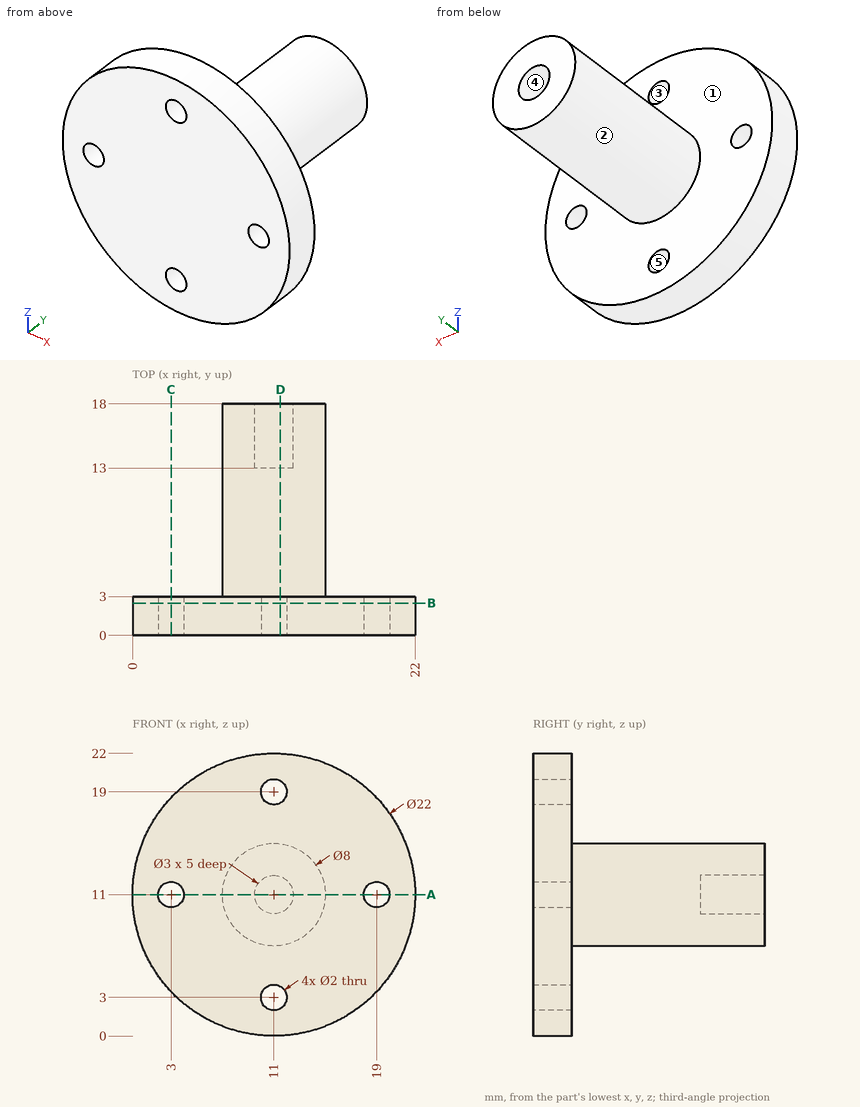
Check sheet for the drawn part. Datum: minimum x, y, z corner. Units: mm. A direction names the side the tool comes from. Round coordinates to 2 decimals unless told otherwise and drop trailing zeros. Loops run counter-clockwise (first coordinate to the right, second up) from the corner with the lowest first, then second, coordinate; pieces in that order, holes last. Notation, with made-up numbers: (7.5, 35) - (63.5, 35) arc R32 cw to (63.5, 67) - close; hole circle Ø5 at (-28.5, -36.75). An arc over 180 degrees is marked (long way). Use one line per item in the form item = value.
1. Section check B-B on y = 2.5. Record the cut outline in (x, z).
A:
outline = circle Ø22 at (11, 11); hole circle Ø2 at (3, 11); hole circle Ø2 at (11, 3); hole circle Ø2 at (11, 19); hole circle Ø2 at (19, 11)
2. Section check C-C on x = 3. Record the cut outline in (y, z), and give its area (3 significant figures).
A:
outline = (0, 3.45) - (3, 3.45) - (3, 10) - (0, 10) - close; (0, 12) - (3, 12) - (3, 18.55) - (0, 18.55) - close
area = 39.3 mm²
3. Section check D-D on x = 11.5. Record the cut outline in (y, z), and give its area (3 significant figures).
A:
outline = (0, 0.01) - (3, 0.01) - (3, 2.13) - (0, 2.13) - close; (0, 3.87) - (3, 3.87) - (3, 7.03) - (18, 7.03) - (18, 9.59) - (13, 9.59) - (13, 12.41) - (18, 12.41) - (18, 14.97) - (3, 14.97) - (3, 18.13) - (0, 18.13) - close; (0, 19.87) - (3, 19.87) - (3, 21.99) - (0, 21.99) - close
area = 160 mm²
4. Draft check along X on the marked faces 1, 2 and 3. Enter one of: pulls with the +X half, pulls with the -X half, needs draft (parallel to the pull), parting line crosses it, or undercut.
A:
face_1 = needs draft
face_2 = parting line crosses it
face_3 = undercut
5. Scan lines: probe 1 along X at (y, z) = (1.8, 11); probe 2 along Y at (x, z) = (12.5, 16); probe 3 along X at (y, z) = (1.5, 19). Record each from-to range of solid material in increasing order.
A:
probe_1 = 0 to 2, 4 to 18, 20 to 22
probe_2 = 0 to 3
probe_3 = 3.45 to 10, 12 to 18.55
6. Gauge pin test, flat ends, axial feed: pin 1 Ø1.5 at (x, z) = (14.5, 4.5) entering from +Y; pin 2 Ø5 at (y, z) = (14, 10.5) entering from -X; pin 3 Ø1.5 at (x, z) = (10.5, 11) entering from +Y. Record the tip position at first contact, or that the pin passes through.
A:
pin_1 = 3
pin_2 = 7
pin_3 = 13
7. Section check A-A on z = 11. Record the cut outline in (x, y).
A:
outline = (0, 0) - (2, 0) - (2, 3) - (0, 3) - close; (4, 0) - (18, 0) - (18, 3) - (15, 3) - (15, 18) - (12.5, 18) - (12.5, 13) - (9.5, 13) - (9.5, 18) - (7, 18) - (7, 3) - (4, 3) - close; (20, 0) - (22, 0) - (22, 3) - (20, 3) - close
8. Access from +Z, -Z, +X, -X, +Y, -Y to the whole of each face (thin tool, end or side, straight path). Record for the marked faces 4 and 5.
A:
face_4 = +Y
face_5 = +Y, -Y
